from build123d import *

# Parameters (mm, degrees)
EXTRUDE_1_DEPTH     = 480
SKETCH_2_R          = 3.5
SKETCH_2_R_2        = 3
CUT_EXTRUDE_1_DEPTH = 481.468521341


with BuildPart() as part:
    # Эскиз1 → Вытянуть-Тонкостенный1 (new body)
    with BuildSketch(Plane(origin=(0, 0, 0), x_dir=(0, 0, -1), z_dir=(1, 0, 0))):
        with BuildLine():
            Line((10, 7.5), (-10, 7.5))
            ThreePointArc((-10, 7.5), (-13.535533906, 6.035533906), (-15, 2.5))
            Line((-15, 2.5), (-15, -2.5))
            ThreePointArc((-15, -2.5), (-13.535533906, -6.035533906), (-10, -7.5))
            Line((-10, -7.5), (10, -7.5))
            ThreePointArc((10, -7.5), (13.535533906, -6.035533906), (15, -2.5))
            Line((15, -2.5), (15, 2.5))
            ThreePointArc((15, 2.5), (13.535533906, 6.035533906), (10, 7.5))
        make_face()
        with BuildLine():
            Line((10, 6.5), (-10, 6.5))
            ThreePointArc((-10, 6.5), (-12.828427125, 5.328427125), (-14, 2.5))
            Line((-14, 2.5), (-14, -2.5))
            ThreePointArc((-14, -2.5), (-12.828427125, -5.328427125), (-10, -6.5))
            Line((-10, -6.5), (10, -6.5))
            ThreePointArc((10, -6.5), (12.828427125, -5.328427125), (14, -2.5))
            Line((14, -2.5), (14, 2.5))
            ThreePointArc((14, 2.5), (12.828427125, 5.328427125), (10, 6.5))
        make_face(mode=Mode.SUBTRACT)
    extrude(amount=EXTRUDE_1_DEPTH)

    # Эскиз2 → Вырез-Вытянуть1 (cut, through all)
    with BuildSketch(Plane(origin=(0, 7.5, 0), x_dir=(1, 0, 0), z_dir=(0, 1, 0))):
        with Locations(Location((240, 0, 0), (0, 0, 270))):
            Circle(SKETCH_2_R)
        with Locations(Location((57.5, 0, 0), (0, 0, 270))):
            Circle(SKETCH_2_R_2)
        with Locations(Location((422.5, 0, 0), (0, 0, 90))):
            Circle(SKETCH_2_R_2)
    extrude(amount=-CUT_EXTRUDE_1_DEPTH, mode=Mode.SUBTRACT)


solid = part.part
The listing builds one solid part. Answer for the finished solid, in the listing's coordinates (mm). Round coordinates to 2 decimals unless told otherwise and drop trailing zeros. Write each loop counter-clockwise with the first axis right and the second up, starting at its lowest first coordinate (ties: lowest second). Pieces come first, ordered by that corner, then holes. Notation, with made-up numbers: M 33.25,29 L 62.25,29 A13 ccw 62.25,40 Z; hole C -10,45.25 d4. An arc over 180 degrees is marked long. Write each question's results on one line, items separated by ' | '. Start each with the question number.
Item 1: A cutting plane is placed at B-B on x = 336. Write down the section's boundary in (y, z).
Item 2: Flat-ended cylindrical pins translate along their axes: pin 1 Ø3 at (x, y) = (240, 6) entering from +Z; pin 2 Ø2 at (y, z) = (0, 12) entering from +X (3 decimals); pin 3 Ø3 at (x, y) = (224, 5.5) entering from +Z. Find the tip coordinate at first contact, or state that the pin passes through.
Item 3: Straight lines are drawn through the part: L1, parallel to X at y = 6.85, z = 0; L2, parallel to Y at x = 171.5, z = 1.5; L3, parallel to Y at x = 242, z = -10.75. For each, find the intervals that lie inside material, in ascending order. Write a range as [from, to].
Item 4: For a pull along Z with two mould halves and no side action, classify faces 1 (the face through (236.6, -7.5, -2.1)), 2 (the face through (236.6, 6.5, 2.1)), 3 (the face through (236.6, -6.5, -2.1)) as pulls with the +Z half, pulls with the -Z half, needs draft (parallel to the pull), parting line crosses it, or undercut.
Item 5: A cutting plane is placed at A-A on y = 0. Write down the section's boundary in (x, z), and give its area (3 significant figures).
Check sheet entries:
1) outline: M -7.5,-10 A5 ccw -2.5,-15 L 2.5,-15 A5 ccw 7.5,-10 L 7.5,10 A5 ccw 2.5,15 L -2.5,15 A5 ccw -7.5,10 Z; hole M -6.5,-10 A4 ccw -2.5,-14 L 2.5,-14 A4 ccw 6.5,-10 L 6.5,10 A4 ccw 2.5,14 L -2.5,14 A4 ccw -6.5,10 Z
2) pin 1: z = 14.58 | pin 2: through | pin 3: z = 14.77
3) L1: [0, 54.5], [60.5, 236.5], [243.5, 419.5], [425.5, 480] | L2: [-7.5, -6.5], [6.5, 7.5] | L3: [-7.44, -6.43], [6.43, 7.44]
4) face 1: needs draft | face 2: undercut | face 3: undercut
5) outline: M 0,-15 L 480,-15 L 480,-14 L 0,-14 Z; M 0,14 L 480,14 L 480,15 L 0,15 Z | area: 960 mm²
